```python
from build123d import *

# Parameters (mm, degrees)
SKETCH2_W           = 10
SKETCH2_H           = 25
BOSS_EXTRUDE1_DEPTH = 5
SKETCH4_W           = 10
SKETCH4_H           = 5
BOSS_EXTRUDE2_DEPTH = 33
SKETCH6_R           = 2
CUT_EXTRUDE1_DEPTH  = 36.640566774
SKETCH7_R           = 2
CUT_EXTRUDE2_DEPTH  = 44.231932642


with BuildPart() as part:
    # Sketch2 → Boss-Extrude1 (new body)
    with BuildSketch(Plane(origin=(0, 0, 0), x_dir=(1, 0, 0), z_dir=(0, 1, 0))):
        Rectangle(SKETCH2_W, SKETCH2_H)
    extrude(amount=BOSS_EXTRUDE1_DEPTH)

    # Sketch4 → Boss-Extrude2 (add)
    with BuildSketch(Plane(origin=(0, 5, 0), x_dir=(1, 0, 0), z_dir=(0, 1, 0))):
        with Locations((0, 10)):
            Rectangle(SKETCH4_W, SKETCH4_H)
    extrude(amount=BOSS_EXTRUDE2_DEPTH)

    # Sketch6 → Cut-Extrude1 (cut, through all)
    with BuildSketch(Plane(origin=(0, 5, 0), x_dir=(1, 0, 0), z_dir=(0, 1, 0))):
        with Locations(Location((0, 2.5, 0), (0, 0, 270))):
            Circle(SKETCH6_R)
        with Locations(Location((0, -7.5, 0), (0, 0, 270))):
            Circle(SKETCH6_R)
    extrude(amount=-CUT_EXTRUDE1_DEPTH, mode=Mode.SUBTRACT)

    # Sketch7 → Cut-Extrude2 (cut, through all)
    with BuildSketch(Plane.XY.offset(-7.5)):
        with Locations((0, 30)):
            Circle(SKETCH7_R)
        with Locations((0, 20)):
            Circle(SKETCH7_R)
    extrude(amount=-CUT_EXTRUDE2_DEPTH, mode=Mode.SUBTRACT)


solid = part.part
```
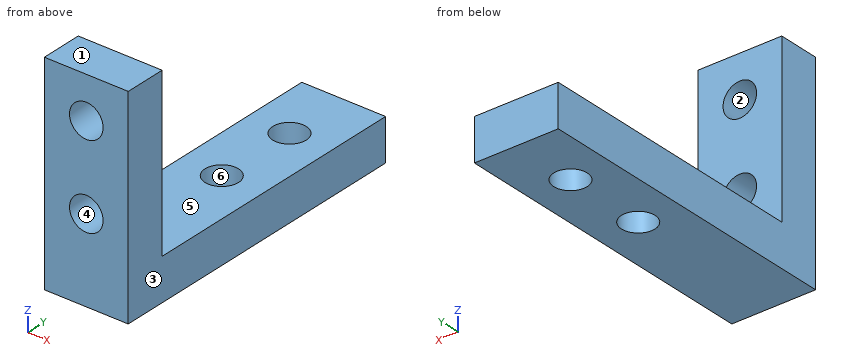
Here's how the part is built. I have some questions about the finished solid (model axes, mm). Face numbers are marked on the shaded views. A direction names the side the tool comes from. Round coordinates to 2 decimals unless told otherwise and drop trailing zeros. Order: outer loops, then holes, each group sorted by start corner. A loop starts at its lowest first (then second) coordinate and runs counter-clockwise, first axis right, second up. Notation, with made-up numbers: M 64,-5 L 99,-5 A31 ccw 99,31 Z; hole C 40,9 d6. An arc over 180 degrees is marked long. Answer in a Markdown table with one row per item.
Item 1: Imagine slicing it at D-D, the plane z = -8. Write out the boundary of the cut face in (x, y).
A:
| item | result |
|---|---|
| outline | M -5,0 L 5,0 L 5,38 L -5,38 Z; hole C 0,20 d4; hole C 0,30 d4 |
Item 2: Thinking about a two-plate mould opening in Z: for the marked faces 1, 2, 3 and 4, which applies, +Z half, -Z half, draft (parallel to the pull), parting line (faces both ways), or undercut?
A:
| item | result |
|---|---|
| face 1 | +Z half |
| face 2 | undercut |
| face 3 | draft |
| face 4 | undercut |
Item 3: For the marked faces 5 and 6, which set-ups out of +Z, -Z, +X, -X, +Y, -Y let a thin tool reach every point of the face, with its end or its side?
A:
| item | result |
|---|---|
| face 5 | +Z, +X, -X, +Y |
| face 6 | +Z, -Z |
Item 4: Imagine slicing it at B-B, the plane z = -2.5. Write out the boundary of the cut face in (x, y).
A:
| item | result |
|---|---|
| outline | M -5,0 L -2,0 L -2,5 L -5,5 Z; M 2,0 L 5,0 L 5,5 L 2,5 Z |
Item 5: Imagine slicing it at A-A, the plane y = 20. Write out the boundary of the cut face in (x, z).
A:
| item | result |
|---|---|
| outline | M -5,-12.5 L -2,-12.5 L -2,-7.5 L -5,-7.5 Z; M 2,-12.5 L 5,-12.5 L 5,-7.5 L 2,-7.5 Z |
Item 6: Imagine slicing it at C-C, the plane x = 0. Write out the boundary of the cut face in (y, z), and give its area (3 significant figures).
A:
| item | result |
|---|---|
| outline | M 0,-12.5 L 18,-12.5 L 18,-7.5 L 5,-7.5 L 5,-4.5 L 0,-4.5 Z; M 0,-0.5 L 5,-0.5 L 5,5.5 L 0,5.5 Z; M 0,9.5 L 5,9.5 L 5,12.5 L 0,12.5 Z; M 22,-12.5 L 28,-12.5 L 28,-7.5 L 22,-7.5 Z; M 32,-12.5 L 38,-12.5 L 38,-7.5 L 32,-7.5 Z |
| area | 210 mm2 |
Item 7: I'm going to push flat-ended pins straight in: pin 1 (5 mm diameter, centred on x = 0, y = 20, fed in from -Z); pin 2 (5 mm diameter, centred on x = 1.5, y = 8.5, fed in from +Z); pin 3 (2.5 mm diameter, centred on x = 0, z = 7.5, fed in from +Y); pin 4 (6 mm diameter, centred on x = 0, z = -3.5, fed in from +Y). Where does each tip first touch, or does it pass through?
A:
| item | result |
|---|---|
| pin 1 | stops at z = -12.5 |
| pin 2 | stops at z = -7.5 |
| pin 3 | passes through |
| pin 4 | stops at y = 5 |
Item 8: If I drill on L1, parallel to Y at x = 0, z = -9.3; L2, parallel to X at y = 3.95, z = 7.5; L3, parallel to Y at x = 3, z = 4.25, over which ranges is the centre line in solid material (lowest first)? Write a range as from..to.
A:
| item | result |
|---|---|
| L1 | y = 0..18, 22..28, 32..38 |
| L2 | x = -5..-2, 2..5 |
| L3 | y = 0..5 |
